For this review, take the finished solid that the model builds, in its own axes (mm). Face numbers are marked on the shaded views. A direction names the side the tool comes from. Give positions to 0.01 mm unless a question says otherwise; leave off trailing zeros. Loops run counter-clockwise (first coordinate to the right, second up) from the corner with the lowest first, then second, coordinate; pieces in that order, holes last.
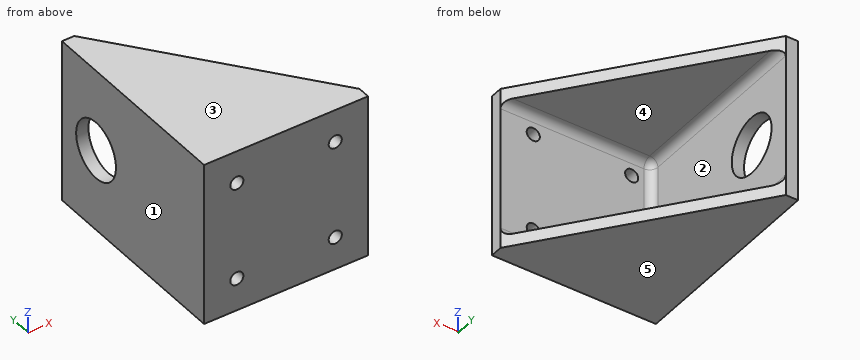
```python
from build123d import *

# Parameters (mm, degrees)
SKETCH3_W           = 40
SKETCH3_H           = 40
SKETCH3_R           = 1.6
BOSS_EXTRUDE2_DEPTH = 3
SKETCH4_W           = 40
SKETCH4_H           = 50
SKETCH4_R           = 7
BOSS_EXTRUDE3_DEPTH = 3
BOSS_EXTRUDE4_DEPTH = 3
FILLET1_R           = 2


with BuildPart() as part:
    # Sketch3 → Boss-Extrude2 (new body)
    with BuildSketch(Plane(origin=(0, 0, 0), x_dir=(1, 0, 0), z_dir=(0, 1, 0))):
        Rectangle(SKETCH3_W, SKETCH3_H)
        with Locations(Location((-12, 12, 0), (0, 0, 270))):
            Circle(SKETCH3_R, mode=Mode.SUBTRACT)
        with Locations(Location((-12, -12, 0), (0, 0, 90))):
            Circle(SKETCH3_R, mode=Mode.SUBTRACT)
        with Locations(Location((12, -12, 0), (0, 0, 270))):
            Circle(SKETCH3_R, mode=Mode.SUBTRACT)
        with Locations(Location((12, 12, 0), (0, 0, 90))):
            Circle(SKETCH3_R, mode=Mode.SUBTRACT)
    extrude(amount=BOSS_EXTRUDE2_DEPTH)

    # Sketch4 → Boss-Extrude3 (add)
    with BuildSketch(Plane.ZY.offset(20)):
        with Locations((0, 25)):
            Rectangle(SKETCH4_W, SKETCH4_H)
        with Locations((0, 38)):
            Circle(SKETCH4_R, mode=Mode.SUBTRACT)
    extrude(amount=-BOSS_EXTRUDE3_DEPTH)

    # Sketch5 → Boss-Extrude4 (add)
    with BuildSketch(Plane.XY.offset(20)):
        Polygon((-20, 50), (-17, 50), (20, 3), (20, 0), (-20, 0), align=None)
    boss_extrude4 = extrude(amount=-BOSS_EXTRUDE4_DEPTH)

    # Mirror1: Boss-Extrude4 across plane
    add(boss_extrude4.mirror(Plane.XY))

    # Fillet1
    fillet1_edges = [part.edges().sort_by_distance(p)[0] for p in [
        (-17, 26.5, 17),
        (1.5, 3, 17),
        (-17, 3, 0),
        (-17, 26.5, -17),
        (1.5, 3, -17),
    ]]
    fillet(fillet1_edges, radius=FILLET1_R)


solid = part.part
```
Item 1: For L1, parallel to X at y = 1.8, z = -12; L2, parallel to Y at x = -18.5, z = 0; L3, parallel to Y at x = 5.5, z = 12, list the stretches that pass through material, from the lowest coordinate up.
Answer:
L1: x = -20 to -13.6, -10.4 to 10.4, 13.6 to 20
L2: y = 0 to 31, 45 to 50
L3: y = 0 to 3
Item 2: Take a section at C-C on x = -12. Give the boundary of the cut face in (y, z).
Answer:
outline: (0, -20) - (43.65, -20) - (43.65, -17) - (5, -17) arc R2 cw to (3, -15) - (3, -13.6) - (0, -13.6) - close; (0, -10.4) - (3, -10.4) - (3, 10.4) - (0, 10.4) - close; (0, 13.6) - (3, 13.6) - (3, 15) arc R2 cw to (5, 17) - (43.65, 17) - (43.65, 20) - (0, 20) - close
Item 3: Take a section at B-B on z = 0. Give the boundary of the cut face in (x, y).
Answer:
outline: (-20, 0) - (20, 0) - (20, 3) - (-15, 3) arc R2 cw to (-17, 5) - (-17, 31) - (-20, 31) - close; (-20, 45) - (-17, 45) - (-17, 50) - (-20, 50) - close
Item 4: Clearance check with flat-ended pins moving along their axes: pin 1 Ø24 at (y, z) = (24, -2) entering from +X; pin 2 Ø16.5 at (x, y) = (4, 24) entering from +Z; pin 3 Ø2 at (x, z) = (-5.5, 15.5) entering from +Y; pin 4 Ø6 at (x, z) = (-3, -6) entering from +Y. State where each tip first meets the part, or that it passes through.
Answer:
pin 1: stops at x = -17
pin 2: stops at z = 20
pin 3: stops at y = 3.68
pin 4: stops at y = 3
Item 5: Tool access review of the marked faces 1 and 2: name each direction out of +Z, -Z, +X, -X, +Y, -Y from which nothing blocks a thin tool from reaching the whole face with its end or side.
Answer:
face 1: +Z, -Z, -X, +Y, -Y
face 2: +X, +Y
Item 6: Take a section at A-A on z = 12. Give the boundary of the cut face in (x, y), and give its area (3 significant figures).
Answer:
outline: (-20, 0) - (-13.6, 0) - (-13.6, 3) - (-15, 3) arc R2 cw to (-17, 5) - (-17, 50) - (-20, 50) - close; (-10.4, 0) - (10.4, 0) - (10.4, 3) - (-10.4, 3) - close; (13.6, 0) - (20, 0) - (20, 3) - (13.6, 3) - close
area: 243 mm2
Item 7: The part is to be moulded in two halves that separate along Z. For the marked faces 3, 4 and 5, say which applies: released by +Z, released by -Z, zero draft, split by the parting line, or undercut.
Answer:
face 3: released by +Z
face 4: undercut
face 5: released by -Z
Item 8: Take a section at D-D on y = 32.5. Give the boundary of the cut face in (x, z).
Answer:
outline: (-20, -20) - (-3.22, -20) - (-3.22, -17) - (-15, -17) arc R2 cw to (-17, -15) - (-17, -4.33) - (-20, -4.33) - close; (-20, 4.33) - (-17, 4.33) - (-17, 15) arc R2 cw to (-15, 17) - (-3.22, 17) - (-3.22, 20) - (-20, 20) - close
